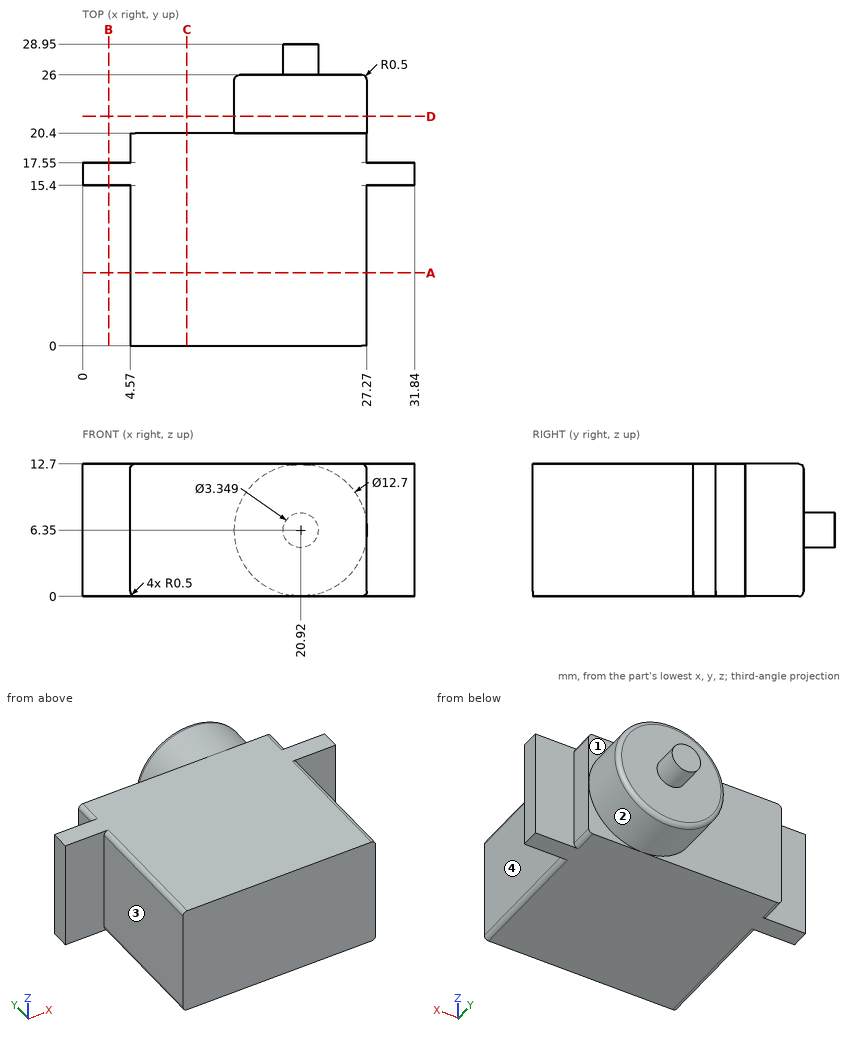
Source: three-view drawing plus pictorial views. Frame: mm from the lowest corner of the part. A direction names the side the tool comes from. Give positions to 0.01 mm unless a question says otherwise; leave off trailing zeros. Loops run counter-clockwise (first coordinate to the right, second up) from the corner with the lowest first, then second, coordinate; pieces in that order, holes last. Notation, with made-up numbers: (-20, 53) -> (-13, 53) arc R22 ccw to (-13, 74) -> close; hole circle Ø6 at (65.25, 27.5). An arc over 180 degrees is marked (long way). Use a Markdown table: item, result. Add a question column.
(1) First-contact query: pin 1 Ø6 at (x, z) = (13.5, 8) entering from +Y; pin 2 Ø5.5 at (x, z) = (29, 4.5) entering from -Y; pin 3 Ø2.5 at (x, z) = (2.5, 6.5) entering from +Y; pin 4 Ø4 at (x, z) = (10, 8.5) entering from +Y. Flat tips, straight axial feed; report the tip coordinate or a pass-through.
(2) Ray query, line 1 (Y direction, x = 20.5, z = 4); line 2 (X direction, y = 19, z = 10.75); line 3 (Y direction, x = 11, z = 5). Return the intervals inside material, ascending.
(3) Section query A-A (y = 7). Output: boundary loops of the cut face in (x, z), then the cut area to 3 significant figures.
(4) Section query D-D (y = 22). Output: boundary loops of the cut face in (x, z).
(5) Section query B-B (x = 2.5). Output: boundary loops of the cut face in (y, z), then the cut area to 3 significant figures.
(6) Access query for the marked faces 1, 2, 3 and 4. Directions: +Z, -Z, +X, -X, +Y, -Y. A direction counts if a zero-diameter tool reaches every point of the face in a straight line with its end or side. Return the directions, or none.
(7) Section query C-C (x = 10). Output: boundary loops of the cut face in (y, z).
Checked values:
| question | item | result |
|---|---|---|
| 1 | pin 1 | y = 26 |
| 1 | pin 2 | y = 0 |
| 1 | pin 3 | y = 17.55 |
| 1 | pin 4 | y = 20.4 |
| 2 | line 1 | 0 to 26 |
| 2 | line 2 | 4.57 to 27.27 |
| 2 | line 3 | 0 to 20.4 |
| 3 | outline | (4.57, 0.5) arc R0.5 ccw to (5.07, 0) -> (26.77, 0) arc R0.5 ccw to (27.27, 0.5) -> (27.27, 12.2) arc R0.5 ccw to (26.77, 12.7) -> (5.07, 12.7) arc R0.5 ccw to (4.57, 12.2) -> close |
| 3 | area | 288 mm^2 |
| 4 | outline | circle Ø12.7 at (20.92, 6.35) |
| 5 | outline | (15.4, 0) -> (17.55, 0) -> (17.55, 12.7) -> (15.4, 12.7) -> close |
| 5 | area | 27.3 mm^2 |
| 6 | face 1 | +Z, +X, +Y |
| 6 | face 2 | +Y |
| 6 | face 3 | +Z, -Z, -X, -Y |
| 6 | face 4 | +Z, -Z, +X, -Y |
| 7 | outline | (0, 0) -> (20.4, 0) -> (20.4, 12.7) -> (0, 12.7) -> close |
